```python
from build123d import *

# Parameters (mm, degrees)
SKETCH1_R           = 2
BOSS_EXTRUDE1_DEPTH = 9.5
SKETCH2_R           = 2
CUT_EXTRUDE1_DEPTH  = 12
SKETCH3_R           = 3.6
CUT_EXTRUDE2_DEPTH  = 4
SKETCH4_R           = 3.6
CUT_EXTRUDE3_DEPTH  = 4


with BuildPart() as part:
    # Sketch1 → Boss-Extrude1 (new body)
    with BuildSketch(Plane.XY):
        Polygon((-4.122741548, -0.104764568), (-12.122741548, -0.104764568), (-56.964364606, -47.160357663), (-56.964364606, -53.160357663), (-10.122741548, -53.160357663), (-4.122741548, -53.160357663), align=None)
        with Locations((-52.622741548, -48.884592163)):
            Circle(SKETCH1_R, mode=Mode.SUBTRACT)
        with Locations((-9.622741548, -10.884592163)):
            Circle(SKETCH1_R, mode=Mode.SUBTRACT)
    extrude(amount=BOSS_EXTRUDE1_DEPTH)

    # Sketch2 → Cut-Extrude1 (cut)
    with BuildSketch(Plane(origin=(-4.122741548, 0, 0), x_dir=(0, 0, -1), z_dir=(1, 0, 0))):
        with Locations((-5, -19.600993214)):
            Circle(SKETCH2_R)
        with Locations((-5, -34.600993214)):
            Circle(SKETCH2_R)
    extrude(amount=-CUT_EXTRUDE1_DEPTH, mode=Mode.SUBTRACT)

    # Sketch3 → Cut-Extrude2 (cut)
    with BuildSketch(Plane.XY.offset(9.5)):
        with Locations((-52.622741548, -48.884592163)):
            Circle(SKETCH3_R)
    extrude(amount=-CUT_EXTRUDE2_DEPTH, mode=Mode.SUBTRACT)

    # Sketch4 → Cut-Extrude3 (cut)
    with BuildSketch(Plane.XY.offset(9.5)):
        with Locations((-9.622741548, -10.884592163)):
            Circle(SKETCH4_R)
    extrude(amount=-CUT_EXTRUDE3_DEPTH, mode=Mode.SUBTRACT)


solid = part.part
```
Geometry check sheet. Reference: the model listing, model coordinates, mm. A direction names the side the tool comes from. Coordinates: 2 decimals unless noted, no trailing zeros. Loops run counter-clockwise (first coordinate to the right, second up) from the corner with the lowest first, then second, coordinate; pieces in that order, holes last. Notation, with made-up numbers: (76, -13.75) - (115, -13.75) arc R21 ccw to (115, 6.25) - close; hole circle Ø2 at (-37.75, 21). An arc over 180 degrees is marked (long way). One line per item, written item: value. Start each with the question number.
(1) Mould release check, pull along X, two halves, no side actions. Record for faces 4 (the flat face through (-8.07, -12.43, 5.5)), 5 (the flat face through (-56.964, -50, 5)), 6 (the cylindrical face through (-6.19, -9.8, 7.53)), 7 (the flat face through (-25, -32, 0)): released by +X, released by -X, zero draft, split by the parting line, or undercut.
(2) Depth check by flat-ended pin: P1, Ø5, axis at x = -9.62, y = -10.88, coming from the +Z side; P2, Ø3.5, axis at y = -19.6, z = 5, coming from the +X side; P3, Ø1, axis at y = -28, z = 1, coming from the -X side. Enter the tip coordinate at first touch or a pass-through.
(3) Cross-section at A-A on x = -53.5. Enter the section's corners in (y, z), plus the area to 3 significant figures.
(4) Cross-section at B-B on y = -25. Enter the section's corners in (x, z).
(5) Material ranges on line 1 (Y direction, x = -7, z = 5); line 2 (Y direction, x = -10.25, z = 5); line 3 (Y direction, x = -10.75, z = 5), recorded low to high. Write a range as [from, to].
(6) Cross-section at C-C on x = -42.5. Enter the section's corners in (y, z), plus the area to 3 significant figures.
(7) Tool access check on faces 1 (the cylindrical face through (-55.276, -46.452, 7.528)), 2 (the cylindrical face through (-10.039, -17.618, 5.26)), 3 (the flat face through (-31, -53.16, 5)). Record the directions out of +Z, -Z, +X, -X, +Y, -Y that give a thin tool (end or side, any length) a straight path to the whole face; none if there is none.
Results below:
1. face 4: undercut
1. face 5: released by -X
1. face 6: undercut
1. face 7: zero draft
2. P1: stops at z = 5.5
2. P2: stops at x = -16.12
2. P3: stops at x = -39.18
3. outline: (-53.16, 0) - (-50.68, 0) - (-50.68, 5.5) - (-52.38, 5.5) - (-52.38, 9.5) - (-53.16, 9.5) - close; (-47.09, 0) - (-43.52, 0) - (-43.52, 9.5) - (-45.39, 9.5) - (-45.39, 5.5) - (-47.09, 5.5) - close
3. area: 43.8 mm2
4. outline: (-35.85, 0) - (-4.12, 0) - (-4.12, 9.5) - (-35.85, 9.5) - close
5. line 1: y = [-53.16, -36.6], [-32.6, -21.6], [-17.6, -0.1]
5. line 2: y = [-53.16, -36.6], [-32.6, -21.6], [-17.6, -12.78], [-8.99, -0.1]
5. line 3: y = [-53.16, -36.6], [-32.6, -21.6], [-17.6, -12.54], [-9.23, -0.1]
6. outline: (-53.16, 0) - (-31.98, 0) - (-31.98, 9.5) - (-53.16, 9.5) - close
6. area: 201 mm2
7. face 1: +Z
7. face 2: +X
7. face 3: +Z, -Z, +X, -X, -Y
